from build123d import *

# Parameters (mm, degrees)
SKETCH1_W                        = 80
SKETCH1_H                        = 80
BOSS_EXTRUDE1_DEPTH              = 30
M56_CLEARANCE_HOLE1_D            = 66
M56_CLEARANCE_HOLE1_DEPTH        = 4.4
SKETCH4_W                        = 3
SKETCH4_H                        = 2
SKETCH5_W                        = 30
SKETCH5_H                        = 2.4
F_10_5_10_5_DIAMETER_HOLE1_D     = 10.5
F_10_5_10_5_DIAMETER_HOLE1_DEPTH = 30
F_10_5_10_5_DIAMETER_HOLE2_D     = 10.5
F_10_5_10_5_DIAMETER_HOLE2_DEPTH = 30
CHAMFER1_SIZE                    = 5
CHAMFER2_SIZE                    = 0.5
CHAMFER3_SIZE                    = 1.2
SCALE1_SCALE                     = 0.75


with BuildPart() as part:
    # Sketch1 → Boss-Extrude1 (new body)
    with BuildSketch(Plane(origin=(0, 0, 0), x_dir=(-1, 0, 0), z_dir=(0, 0, -1))):
        Rectangle(SKETCH1_W, SKETCH1_H)
    extrude(amount=-BOSS_EXTRUDE1_DEPTH)

    # M56 Clearance Hole1
    with Locations(Plane(origin=(0, 0, 0), x_dir=(-1, 0, 0), z_dir=(0, 0, -1))):
        with Locations((0, 0)):
            Hole(M56_CLEARANCE_HOLE1_D / 2, depth=M56_CLEARANCE_HOLE1_DEPTH)

    # Sketch4 → Cut-Revolve1 (revolve, cut)
    with BuildSketch(Plane.XZ):
        with Locations((34.5, 1)):
            Rectangle(SKETCH4_W, SKETCH4_H)
    revolve(axis=Axis((0, 0, 2), (0, 0, -1)), mode=Mode.SUBTRACT)

    # Sketch5 → Revolve1 (revolve)
    with BuildSketch(Plane.XZ):
        with Locations((15, 3.2)):
            Rectangle(SKETCH5_W, SKETCH5_H)
    revolve(axis=Axis((0, 0, 4.4), (0, 0, -1)))

    # Sketch6 → Cut-Revolve2 (revolve, cut)
    with BuildSketch(Plane.XZ):
        Polygon((16, 30), (0, 30), (0, 2), (26, 2), (26, 17), (22, 17), (22, 18), (16, 18), (16, 20.738804844), (20, 22), (20, 26), (16, 27.261195156), align=None)
    revolve(axis=Axis((0, 0, 30), (0, 0, -1)), mode=Mode.SUBTRACT)

    # Ø10.5 (10.5) Diameter Hole1
    with Locations(Plane.XY.offset(30)):
        with Locations((-30, -30), (30, 30)):
            Hole(F_10_5_10_5_DIAMETER_HOLE1_D / 2, depth=F_10_5_10_5_DIAMETER_HOLE1_DEPTH)

    # Ø10.5 (10.5) Diameter Hole2
    with Locations(Plane(origin=(0, 0, 0), x_dir=(-1, 0, 0), z_dir=(0, 0, -1))):
        with Locations((30, 30), (-30, -30)):
            Hole(F_10_5_10_5_DIAMETER_HOLE2_D / 2, depth=F_10_5_10_5_DIAMETER_HOLE2_DEPTH)

    # Chamfer1
    chamfer1_edges = [part.edges().sort_by_distance(p)[0] for p in [
        (-40, -40, 15),
        (40, -40, 15),
        (40, 40, 15),
        (-40, 40, 15),
    ]]
    chamfer(chamfer1_edges, length=CHAMFER1_SIZE)

    # Chamfer2
    chamfer2_edges = [part.edges().sort_by_distance(p)[0] for p in [
        (35.25, 30, 30),
        (35.25, 30, 0),
        (-24.75, -30, 30),
        (-24.75, -30, 0),
        (24.75, -30, 0),
        (24.75, -30, 30),
        (-35.25, 30, 0),
        (-35.25, 30, 30),
    ]]
    chamfer(chamfer2_edges, length=CHAMFER2_SIZE)

    # Chamfer3
    chamfer3_edges = [part.edges().sort_by_distance(p)[0] for p in [
        (-26, 0, 2),
    ]]
    chamfer(chamfer3_edges, length=CHAMFER3_SIZE)


with BuildPart() as part_1:
    # Scale1: scaled about (0, 0, 16.565087269)
    add(part.part.scale(SCALE1_SCALE).moved(Location((0, 0, 4.141271817))))


solid = part_1.part
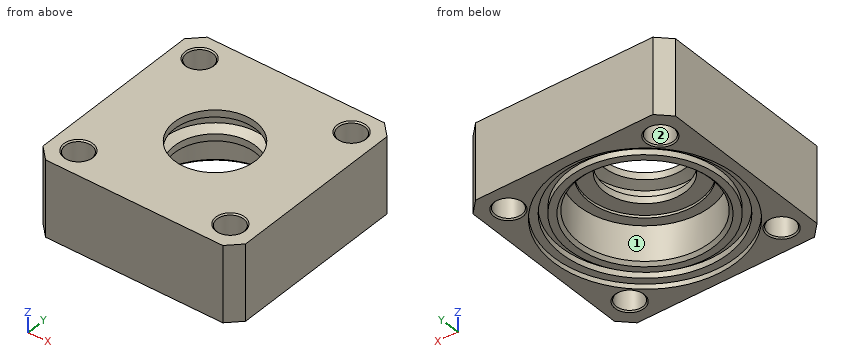
Read the model definition and answer for the solid it produces. Units are mm, in the model's axes. Face numbers are marked on the shaded views. A direction names the side the tool comes from. Give positions to 0.01 mm unless a question says otherwise; leave off trailing zeros. Use a Markdown table: item, result.
Q1. Each of these flat-tipped pins is pushed along its axis until it touches: pin 1 (22.5 mm diameter, centred on x = 7, y = -8, fed in from -Z); pin 2 (6 mm diameter, centred on x = -11.5, y = -7, fed in from -Z). Where does it stop, or does it pass through?
Solved:
| item | result |
|---|---|
| pin 1 | stops at z = 5.64 |
| pin 2 | stops at z = 17.64 |
Q2. Find the intervals of material crossed by line 1 along X through (y, z) = (0, 6.7); line 2 along Y through (x, z) = (-6, 10.5); line 3 along Y through (x, z) = (25, 20.5), in increasing order.
Solved:
| item | result |
|---|---|
| line 1 | x = -30 to -24.75, -22.5 to -19.5, 19.5 to 22.5, 24.75 to 30 |
| line 2 | y = -30 to -18.55, 18.55 to 30 |
| line 3 | y = -30 to -25.54, -19.46 to 19.46, 25.54 to 30 |
Q3. Section A-A, the plane z = 9.5 is taken. Count the separate pieces of the cut face and the enclosed holes in it, then the cut area to 3 significant figures.
Solved:
| item | result |
|---|---|
| separate pieces | 1 |
| enclosed holes | 5 |
| area | 2,180 mm^2 |
Q4. A tool of negligible diameter and unlimited length cuts with its end or side. For the marked faces 1 and 2, from which of +Z, -Z, +X, -X, +Y, -Y can it reach the whole face along a straight path? Write none if from no direction.
Solved:
| item | result |
|---|---|
| face 1 | -Z |
| face 2 | +Z, -Z |
